Can you work these out from the drawing? Everything is in mm from the part's minimum corner. A direction names the side the tool comes from. Coordinates: 2 decimals unless noted, no trailing zeros. Write each loop counter-clockwise with the first axis right and the second up, starting at its lowest first coordinate (ties: lowest second). Pieces come first, ordered by that corner, then holes.
(1) Imagine slicing it at A-A, the plane z = 17. List the corners of the cut face in (x, y) for me.
(2) Please list where these lines run through material, in increasing order: probe 1 along Z at (x, y) = (22.25, 8); probe 2 along Z at (x, y) = (9.5, 2.75) (1 decimal); probe 3 along X at (y, z) = (1, 12) (1 decimal).
(3) Thinking about a two-plate mould opening in Z: for the marked faces 4, 5 and 6, which applies, released by +Z, released by -Z, zero draft, split by the parting line, or undercut?
(4) Which directions (+Z, -Z, +X, -X, +Y, -Y) give clear straight access to the entire face, cutting with the end or side of a thin tool? Please do the marked faces 1, 2 and 3.
(5) Imagine slicing it at B-B, the plane x = 5.5. List the corners of the cut face in (y, z) for me (1 decimal).
(6) Imagine slicing it at C-C, the plane y = 3.75. List the corners of the cut face in (x, z) for me (1 decimal), plus the area to 3 significant figures.
(7) For pin 1 Ø1.5 at (y, z) = (8, 6.5) entering from -X (1 decimal); pin 2 Ø12 at (x, z) = (11, 20.5) entering from -Y; pin 3 Ø5 at (x, y) = (22.5, 3) entering from -Z; pin 4 Ø4 at (x, y) = (15.5, 6) entering from -Z, each with a flat end and sliding along its axis, tell me the tip position at first contact or that it passes through.
(8) Imagine slicing it at D-D, the plane z = 10. List the corners of the cut face in (x, y) for me, plus the area to 3 significant figures.
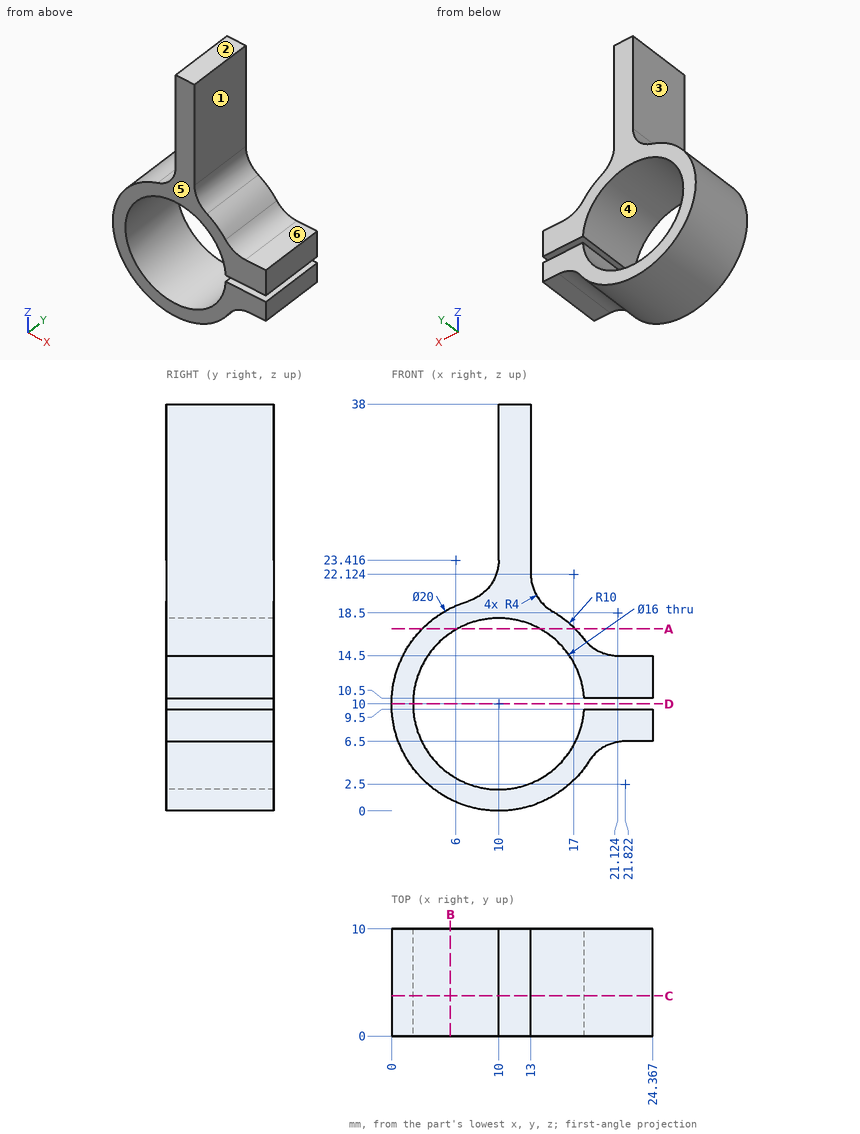
Recorded:
1. outline: (2.86, 0) - (6.13, 0) - (6.13, 10) - (2.86, 10) - close; (13.87, 0) - (17.14, 0) - (17.14, 10) - (13.87, 10) - close
2. probe 1: z = 6.5 to 9.5, 10.5 to 14.5
2. probe 2: z = 0 to 2, 18 to 21.5
2. probe 3: x = 0.2 to 2.3, 17.7 to 24.4
3. face 4: undercut
3. face 5: zero draft
3. face 6: released by +Z
4. face 1: +Z, +X, +Y, -Y
4. face 2: +Z, +X, -X, +Y, -Y
4. face 3: +Z, -X, +Y, -Y
5. outline: (0, 1.1) - (10, 1.1) - (10, 3.4) - (0, 3.4) - close; (0, 16.6) - (10, 16.6) - (10, 18.9) - (0, 18.9) - close
6. outline: (7.1, 19.6) arc R10 ccw (long way) to (18.4, 4.6) arc R4 cw to (21.8, 6.5) - (24.4, 6.5) - (24.4, 9.5) - (18, 9.5) arc R8 cw (long way) to (18, 10.5) - (24.4, 10.5) - (24.4, 14.5) - (21.1, 14.5) arc R4 cw to (17.9, 16.1) arc R10 ccw to (15, 18.7) arc R4 cw to (13, 22.1) - (13, 38) - (10, 38) - (10, 23.4) arc R4 cw to start
6. area: 203 mm2
7. pin 1: stops at x = 0.4
7. pin 2: stops at y = 0
7. pin 3: stops at z = 6.06
7. pin 4: stops at z = 0.63
8. outline: (0, 0) - (2, 0) - (2, 10) - (0, 10) - close
8. area: 20.0 mm2
